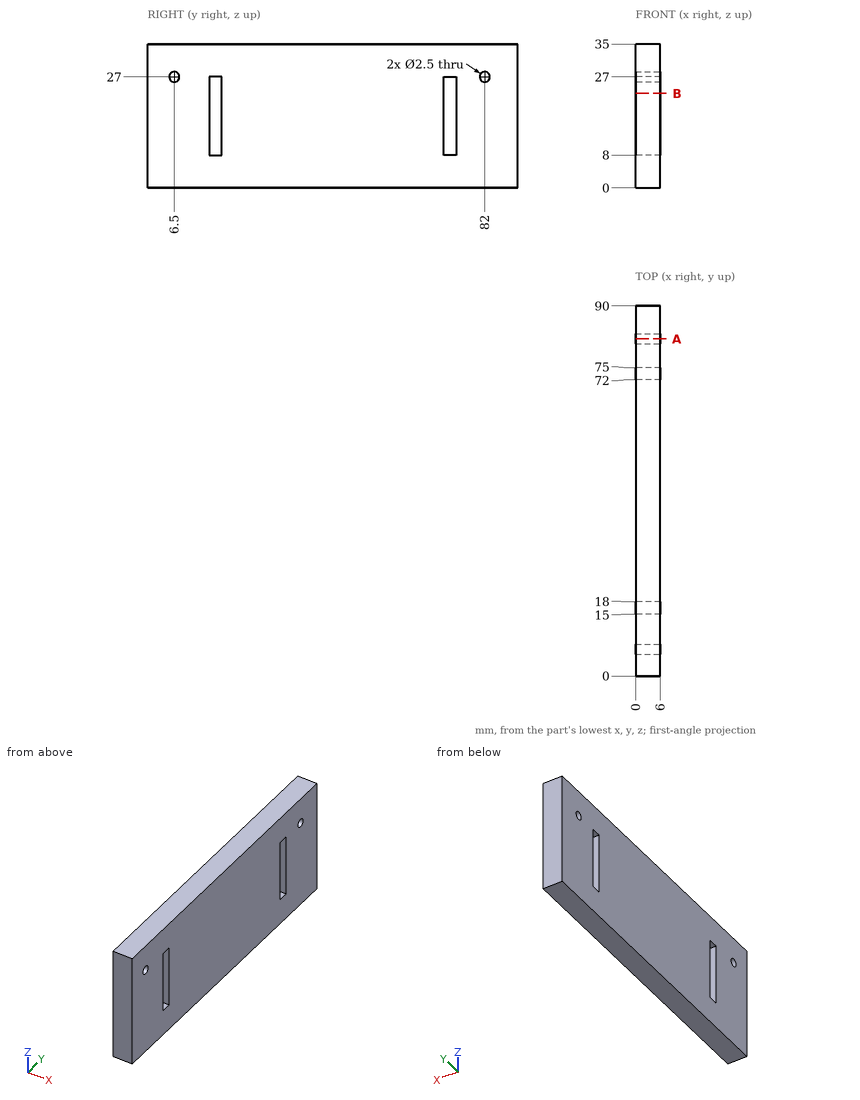
Design review of the part shown in the three views and the two pictorial views. Dimensions are in mm from the part's minimum x, y and z. Round coordinates to 2 decimals unless told otherwise and drop trailing zeros. Loops run counter-clockwise (first coordinate to the right, second up) from the corner with the lowest first, then second, coordinate; pieces in that order, holes last. Notation, with made-up numbers: (3.5, 33.5) - (15.5, 33.5) arc R29 ccw to (15.5, 60.5) - close; hole circle Ø6 at (-36, 72.25). An arc over 180 degrees is marked (long way). Write each question's results on one line, items separated by ' | '. Start each with the question number.
Q1. Wall thickness on line 1 along Y through (x, z) = (4.7, 8.5); line 2 along Z through (x, y) = (4.4, 82); line 3 along Z through (x, y) = (2.6, 72.5): over which ranges is each line inside the solid? List them lowest first. Write a range as [from, to].
Q2. Take a section at A-A on y = 82. Give the boundary of the cut face in (x, z), plus the area to 3 significant figures.
Q3. Take a section at B-B on z = 23. Give the boundary of the cut face in (x, y).
Q4. Insertion check: P1, Ø2, axis at y = 67, z = 22.5, coming from the -X side; P2, Ø2, axis at y = 6.5, z = 27, coming from the +X side. Each pin has a flat end and moves straight along its axis. Give the tip position at first contact, or say it passes through.
Data:
1) line 1: y = [0, 15], [18, 72], [75, 90] | line 2: z = [0, 25.75], [28.25, 35] | line 3: z = [0, 8], [27, 35]
2) outline: (0, 0) - (6, 0) - (6, 25.75) - (0, 25.75) - close; (0, 28.25) - (6, 28.25) - (6, 35) - (0, 35) - close | area: 195 mm²
3) outline: (0, 0) - (6, 0) - (6, 15) - (0, 15) - close; (0, 18) - (6, 18) - (6, 72) - (0, 72) - close; (0, 75) - (6, 75) - (6, 90) - (0, 90) - close
4) P1: stops at x = 0 | P2: passes through
